Read the model definition and answer for the solid it produces. Units are mm, in the model's axes. Face numbers are marked on the shaded views. A direction names the side the tool comes from. Coordinates: 2 decimals unless noted, no trailing zeros. Order: outer loops, then holes, each group sorted by start corner. A loop starts at its lowest first (then second) coordinate and runs counter-clockwise, first axis right, second up. Notation, with made-up numbers: M 58.5,49 L 93.5,49 A19 cw 93.5,86 Z; hole C 63,27 d7. An arc over 180 degrees is marked long. One line per question, with ' | ' between items. Start each with the question number.
1) A tool of negligible diameter and unlimited length cuts with its end or side. For the marked faces 5, 6, 7, 8 and 9, from which of +Z, -Z, +X, -X, +Y, -Y can it reach the whole face along a straight path? Write none if from no direction.
2) The mould has two halves that part along Y. Classify the marked faces 1, 2, 3 and 4: +Y half, -Y half, draft (parallel to the pull), parting line (faces both ways), or undercut.
3) Find section D-D, the plane x = 32.5. Write down the section's boundary in (y, z).
4) Find section C-C, the plane z = 2. Write down the section's boundary in (x, y) (3 decimals), plus the area to 3 significant figures.
5) Find section A-A, the plane z = 18.5. Write down the section's boundary in (x, y) (3 decimals), plus the area to 3 significant figures.
6) Given P1, Ø1.5, axis at x = 13.5, z = 18.5, coming from the -Y side; P2, Ø12, axis at x = 12.5, z = 21, coming from the +Y side; P3, Ø4, axis at x = 16.5, z = 4, coming from the +Y side, each flat-ended and moving along its own axis, determine where each tip first touches the part or whether it passes through.
7) Find section B-B, the plane y = 5.5. Write down the section's boundary in (x, z).
8) Consider probe 1 along Z at (x, y) = (11.5, 12.25); probe 2 along X at (y, z) = (26.75, 8.5); probe 3 along X at (y, z) = (9, 13.75). Determine where each line is inside the solid, lowest interval first.
from build123d import *

# Parameters (mm, degrees)
BOSS_EXTRUDE2_DEPTH = 30
CUT_EXTRUDE1_START  = -5
SKETCH4_R           = 18.5
SKETCH4_R_2         = 7.45
CUT_EXTRUDE1_DEPTH  = 20


with BuildPart() as part:
    # Sketch1 → Boss-Extrude2 (new body)
    with BuildSketch(Plane.XY):
        with BuildLine():
            ThreePointArc((0, 1), (0.292893219, 0.292893219), (1, 0))
            Line((1, 0), (5.75, 0))
            ThreePointArc((5.75, 0), (6.457106781, 0.292893219), (6.75, 1))
            Line((6.75, 1), (6.75, 1.906613378))
            Line((6.75, 1.906613378), (17.725, 7.191778867))
            ThreePointArc((17.725, 7.191778867), (13.3, 14), (17.725, 20.808221133))
            Line((17.725, 20.808221133), (6.75, 26.093386622))
            Line((6.75, 26.093386622), (6.75, 27))
            ThreePointArc((6.75, 27), (6.457106781, 27.707106781), (5.75, 28))
            Line((5.75, 28), (1, 28))
            ThreePointArc((1, 28), (0.292893219, 27.707106781), (0, 27))
            Line((0, 27), (0, 1))
        make_face()
        with BuildLine():
            ThreePointArc((17.725, 20.808221133), (13.3, 14), (17.725, 7.191778867))
            ThreePointArc((17.725, 7.191778867), (20.75, 6.55), (23.775, 7.191778867))
            ThreePointArc((23.775, 7.191778867), (26.996549047, 9.940058498), (28.2, 14))
            ThreePointArc((28.2, 14), (26.996549047, 18.059941502), (23.775, 20.808221133))
            ThreePointArc((23.775, 20.808221133), (20.75, 21.45), (17.725, 20.808221133))
        make_face()
        with BuildLine():
            ThreePointArc((28.2, 14), (26.996549047, 9.940058498), (23.775, 7.191778867))
            Line((23.775, 7.191778867), (34.75, 1.906613378))
            Line((34.75, 1.906613378), (34.75, 1))
            ThreePointArc((34.75, 1), (35.042893219, 0.292893219), (35.75, 0))
            Line((35.75, 0), (40.5, 0))
            ThreePointArc((40.5, 0), (41.207106781, 0.292893219), (41.5, 1))
            Line((41.5, 1), (41.5, 27))
            ThreePointArc((41.5, 27), (41.207106781, 27.707106781), (40.5, 28))
            Line((40.5, 28), (35.75, 28))
            ThreePointArc((35.75, 28), (35.042893219, 27.707106781), (34.75, 27))
            Line((34.75, 27), (34.75, 26.093386622))
            Line((34.75, 26.093386622), (23.775, 20.808221133))
            ThreePointArc((23.775, 20.808221133), (26.996549047, 18.059941502), (28.2, 14))
        make_face()
    extrude(amount=BOSS_EXTRUDE2_DEPTH)

    # Sketch4 → Cut-Extrude1 (cut)
    with BuildSketch(Plane(origin=(0, 0, 0), x_dir=(-1, 0, 0), z_dir=(0, 0, -1)).offset(CUT_EXTRUDE1_START)):
        with Locations((-20.75, 14)):
            Circle(SKETCH4_R)
        with Locations(Location((-20.75, 14, 0), (0, 0, 293.956332154))):
            Circle(SKETCH4_R_2, mode=Mode.SUBTRACT)
    extrude(amount=-CUT_EXTRUDE1_DEPTH, mode=Mode.SUBTRACT)


solid = part.part
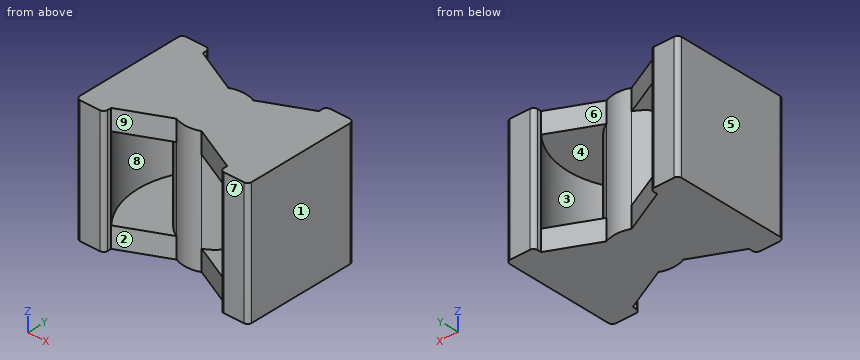
Report:
1) face 5: +Z, -Z, -X, +Y, -Y | face 6: +Z, -Z, +Y | face 7: +Z, -Z, +X, -X, -Y | face 8: none | face 9: +Z, -Z, -Y
2) face 1: draft | face 2: -Y half | face 3: undercut | face 4: undercut
3) outline: M 2.99,0 L 25.01,0 L 25.01,5 L 2.99,5 Z; M 2.99,25 L 25.01,25 L 25.01,30 L 2.99,30 Z
4) outline: M 0,1 A1 ccw 1,0 L 5.75,0 A1 ccw 6.75,1 L 6.75,1.907 L 17.725,7.192 A7.45 ccw 23.775,7.192 L 34.75,1.907 L 34.75,1 A1 ccw 35.75,0 L 40.5,0 A1 ccw 41.5,1 L 41.5,27 A1 ccw 40.5,28 L 35.75,28 A1 ccw 34.75,27 L 34.75,26.093 L 23.775,20.808 A7.45 ccw 17.725,20.808 L 6.75,26.093 L 6.75,27 A1 ccw 5.75,28 L 1,28 A1 ccw 0,27 Z | area: 879 mm^2
5) outline: M 0,1 A1 ccw 1,0 L 5.75,0 A1 ccw 6.75,1 L 6.75,1.907 A18.5 cw 6.75,26.093 L 6.75,27 A1 ccw 5.75,28 L 1,28 A1 ccw 0,27 Z; C 20.75,14 d14.9; M 34.75,1 A1 ccw 35.75,0 L 40.5,0 A1 ccw 41.5,1 L 41.5,27 A1 ccw 40.5,28 L 35.75,28 A1 ccw 34.75,27 L 34.75,26.093 A18.5 cw 34.75,1.907 Z | area: 402 mm^2
6) P1: stops at y = 10.36 | P2: stops at y = 27.66 | P3: stops at y = 22.36
7) outline: M 0,0 L 14.21,0 L 14.21,5 L 4.32,5 L 4.32,25 L 14.21,25 L 14.21,30 L 0,30 Z; M 27.29,0 L 41.5,0 L 41.5,30 L 27.29,30 L 27.29,25 L 37.18,25 L 37.18,5 L 27.29,5 Z
8) probe 1: z = 0 to 5, 25 to 30 | probe 2: x = 0 to 6.75, 34.75 to 41.5 | probe 3: x = 0 to 2.94, 15.23 to 26.27, 38.56 to 41.5
